Read the model definition and answer for the solid it produces. Units are mm, in the model's axes. Face numbers are marked on the shaded views. A direction names the side the tool comes from. Round coordinates to 2 decimals unless told otherwise and drop trailing zeros. Loops run counter-clockwise (first coordinate to the right, second up) from the corner with the lowest first, then second, coordinate; pieces in that order, holes last. Notation, with made-up numbers: (-23, 42.5) - (-4, 42.5) arc R30 ccw to (-4, 73.5) - close; hole circle Ø7 at (83.5, 5). An arc over 180 degrees is marked (long way). Answer as CSV lines item,"result".
```python
from build123d import *

# Parameters (mm, degrees)
F0_R     = 31.5
F1_DEPTH = 2.5
F2_R     = 21.5
F3_DEPTH = 3
F4_SIZE2 = 1
F4_SIZE  = 2.9
F5_R     = 2.6
F6_DEPTH = 5.5
F8_COUNT = 6
F7_R     = 12.5
F9_DEPTH = 3
F10_SIZE = 0.5


with BuildPart() as f1:
    # F0 (on Top) → F1 (new body)
    with BuildSketch(Plane.XY):
        Circle(F0_R)
    extrude(amount=F1_DEPTH)

    # F2 (on face) → F3 (join)
    with BuildSketch(Plane.XY.offset(2.5)):
        Circle(F2_R)
    extrude(amount=F3_DEPTH)

    # F4
    f4_edges = [f1.edges().sort_by_distance(p)[0] for p in [
        (-31.5, 0, 2.5),
    ]]
    f4_side = f1.faces().sort_by_distance((-30.609045, 0, 2.5))[0]
    chamfer(f4_edges, length=F4_SIZE, length2=F4_SIZE2, reference=f4_side)

    # F5 (on face) → F6 (cut, through all)
    with BuildSketch(Plane.XY.offset(5.5)):
        with Locations((0, 17)):
            Circle(F5_R)
    f6 = extrude(amount=-F6_DEPTH, mode=Mode.SUBTRACT)

    # F8: F6 ×6 about axis
    f8_axis = Axis((0, 0, 5.5), (0, 0, 1))
    for i in range(1, F8_COUNT):
        add(f6.rotate(f8_axis, i * 360 / F8_COUNT), mode=Mode.SUBTRACT)

    # F7 (on face) → F9 (cut)
    with BuildSketch(Plane.XY.offset(5.5)):
        Circle(F7_R)
    extrude(amount=-F9_DEPTH, mode=Mode.SUBTRACT)

    # F10
    f10_edges = [f1.edges().sort_by_distance(p)[0] for p in [
        (-21.5, 0, 5.5),
    ]]
    chamfer(f10_edges, length=F10_SIZE)


solid = f1.part
```
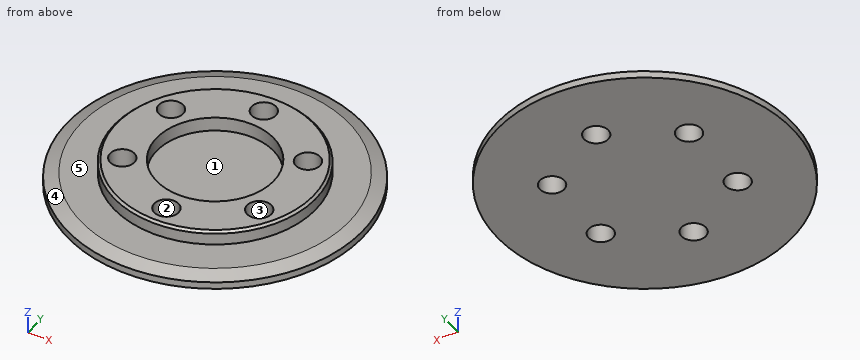
1) A cutting plane is placed at A-A, the plane x = 0. Determine the outline of the cut face in (y, z).
Entries:
outline,"(-31.5, 0) - (-19.6, 0) - (-19.6, 5.5) - (-21, 5.5) - (-21.5, 5) - (-21.5, 2.5) - (-28.6, 2.5) - (-31.5, 1.5) - close; (-14.4, 0) - (14.4, 0) - (14.4, 5.5) - (12.5, 5.5) - (12.5, 2.5) - (-12.5, 2.5) - (-12.5, 5.5) - (-14.4, 5.5) - close; (19.6, 0) - (31.5, 0) - (31.5, 1.5) - (28.6, 2.5) - (21.5, 2.5) - (21.5, 5) - (21, 5.5) - (19.6, 5.5) - close"
2) A cutting plane is placed at C-C, the plane y = -8.5. Count the separate pieces of the cut face and the enclosed holes in it, plus the area to 3 significant figures.
Entries:
separate pieces,"3"
enclosed holes,"0"
area,"155 mm^2"
3) A cutting plane is placed at B-B, the plane y = 0. Determine the outline of the cut face in (x, z), plus the area to 3 significant figures.
Entries:
outline,"(-31.5, 0) - (31.5, 0) - (31.5, 1.5) - (28.6, 2.5) - (21.5, 2.5) - (21.5, 5) - (21, 5.5) - (12.5, 5.5) - (12.5, 2.5) - (-12.5, 2.5) - (-12.5, 5.5) - (-21, 5.5) - (-21.5, 5) - (-21.5, 2.5) - (-28.6, 2.5) - (-31.5, 1.5) - close"
area,"208 mm^2"
4) Each of these flat-tipped pins is pushed along its axis until it touches: P1, Ø5, axis at x = -24.5, y = 19.5, coming from the +Z side; P2, Ø1.5, axis at x = 4.5, z = 3.5, coming from the +Y side. Where does it stop, or does it pass through?
Entries:
P1,"stops at z = 2.43"
P2,"stops at y = 21.17"
5) Find the intervals of material crossed by line 1 (Y direction, x = 0, z = 3.1); line 2 (Y direction, x = 13.5, z = 3.3); line 3 (Z direction, x = 15, y = 18), in increasing order.
Entries:
line 1,"y = -21.5 to -19.6, -14.4 to -12.5, 12.5 to 14.4, 19.6 to 21.5"
line 2,"y = -16.73 to -10.79, -6.21 to 6.21, 10.79 to 16.73"
line 3,"z = 0 to 2.5"
6) The mould has two halves that part along Y. Classify the marked faces 3, 4 and 5: pulls with the +Y half, pulls with the -Y half, needs draft (parallel to the pull), parting line crosses it, or undercut.
Entries:
face 3,"undercut"
face 4,"parting line crosses it"
face 5,"needs draft"
7) A tool of negligible diameter and unlimited length cuts with its end or side. For the marked faces 1 and 2, from which of +Z, -Z, +X, -X, +Y, -Y can it reach the whole face along a straight path? Write none if from no direction.
Entries:
face 1,"+Z"
face 2,"+Z, -Z"
